```python
from build123d import *

# Parameters (mm, degrees)
F0_R     = 1.5
F1_DEPTH = 3
F2_R     = 4.5
F3_DEPTH = 5.2
F4_R     = 1.5
F5_DEPTH = 20


with BuildPart() as f1:
    # F0 (on Front) → F1 (new body)
    with BuildSketch(Plane.XZ):
        with BuildLine():
            Line((5.9394528039, 2.640625), (2.9697264019, 9.3203125))
            ThreePointArc((2.9697264019, 9.3203125), (0, 11.25), (-2.9697264019, 9.3203125))
            Line((-2.9697264019, 9.3203125), (-5.9394528039, 2.640625))
            ThreePointArc((-5.9394528039, 2.640625), (0, -6.5), (5.9394528039, 2.640625))
        make_face()
        with Locations((0, 8)):
            Circle(F0_R, mode=Mode.SUBTRACT)
    extrude(amount=-F1_DEPTH)

    # F2 (on face) → F3 (join)
    with BuildSketch(Plane.XZ):
        Circle(F2_R)
    extrude(amount=F3_DEPTH)

    # F4 (on face) → F5 (join)
    with BuildSketch(Plane.XZ.offset(5.2)):
        Circle(F4_R)
    extrude(amount=F5_DEPTH)


solid = f1.part
```
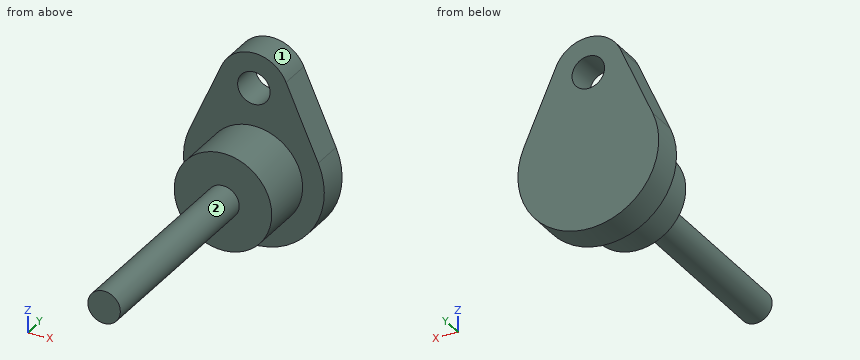
Check sheet for the modelled part. Datum: model origin and axes. Units: mm. Face numbers are marked on the shaded views. A direction names the side the tool comes from. Coordinates: 2 decimals unless noted, no trailing zeros. Order: outer loops, then holes, each group sorted by start corner. A loop starts at its lowest first (then second) coordinate and runs counter-clockwise, first axis right, second up. Notation, with made-up numbers: (-32.75, 62.5) -> (-12.75, 62.5) arc R18 cw to (-12.75, 71.5) -> close; hole circle Ø6 at (-2.75, 82). An arc over 180 degrees is marked (long way). Write each question's results on one line, items separated by ' | '. Start each with the question number.
1) Section check A-A (x = 0). Enter the section's corners in (y, z).
2) Set-up check for the marked faces 1 and 2: record each of +Z, -Z, +X, -X, +Y, -Y from which the full face is reachable in a straight line by a thin tool's end or side.
3) Depth check by flat-ended pin: pin 1 (5 mm diameter, centred on x = 2, y = -21, fed in from -Z); pin 2 (3 mm diameter, centred on y = -16.5, z = 2.5, fed in from +X); pin 3 (6 mm diameter, centred on x = -2.5, y = -12, fed in from +Z); pin 4 (1.8 mm diameter, centred on x = 0, z = 8, fed in from +Y). Enter the tip coordinate at first touch or a pass-through.
4) Section check B-B (z = 0). Enter the section's corners in (x, y), and give its area (3 significant figures).
5) Section check D-D (y = 1.25). Enter the section's corners in (x, z), and give its area (3 significant figures).
6) Material ranges on line 1 along Z through (x, y) = (0, 1.95); line 2 along Y through (x, z) = (4.5, -1.25); line 3 along Y through (x, z) = (3.5, 2.75), recorded low to high.
7) Section check C-C (z = 8). Enter the section's corners in (x, y), and give its area (3 significant figures).
Checked values:
1) outline: (-25.2, -1.5) -> (-5.2, -1.5) -> (-5.2, -4.5) -> (0, -4.5) -> (0, -6.5) -> (3, -6.5) -> (3, 6.5) -> (0, 6.5) -> (0, 4.5) -> (-5.2, 4.5) -> (-5.2, 1.5) -> (-25.2, 1.5) -> close; (0, 9.5) -> (3, 9.5) -> (3, 11.25) -> (0, 11.25) -> close
2) face 1: +Z, +Y, -Y | face 2: -Y
3) pin 1: z = -1.5 | pin 2: x = 1.12 | pin 3: z = 1.5 | pin 4: through
4) outline: (-6.5, 0) -> (-4.5, 0) -> (-4.5, -5.2) -> (-1.5, -5.2) -> (-1.5, -25.2) -> (1.5, -25.2) -> (1.5, -5.2) -> (4.5, -5.2) -> (4.5, 0) -> (6.5, 0) -> (6.5, 3) -> (-6.5, 3) -> close | area: 146 mm²
5) outline: (-5.94, 2.64) arc R6.5 ccw (long way) to (5.94, 2.64) -> (2.97, 9.32) arc R3.25 ccw to (-2.97, 9.32) -> close; hole circle Ø3 at (0, 8) | area: 160 mm²
6) line 1: -6.5 to 6.5, 9.5 to 11.25 | line 2: 0 to 3 | line 3: -5.2 to 3
7) outline: (-3.56, 0) -> (-1.5, 0) -> (-1.5, 3) -> (-3.56, 3) -> close; (1.5, 0) -> (3.56, 0) -> (3.56, 3) -> (1.5, 3) -> close | area: 12.3 mm²
